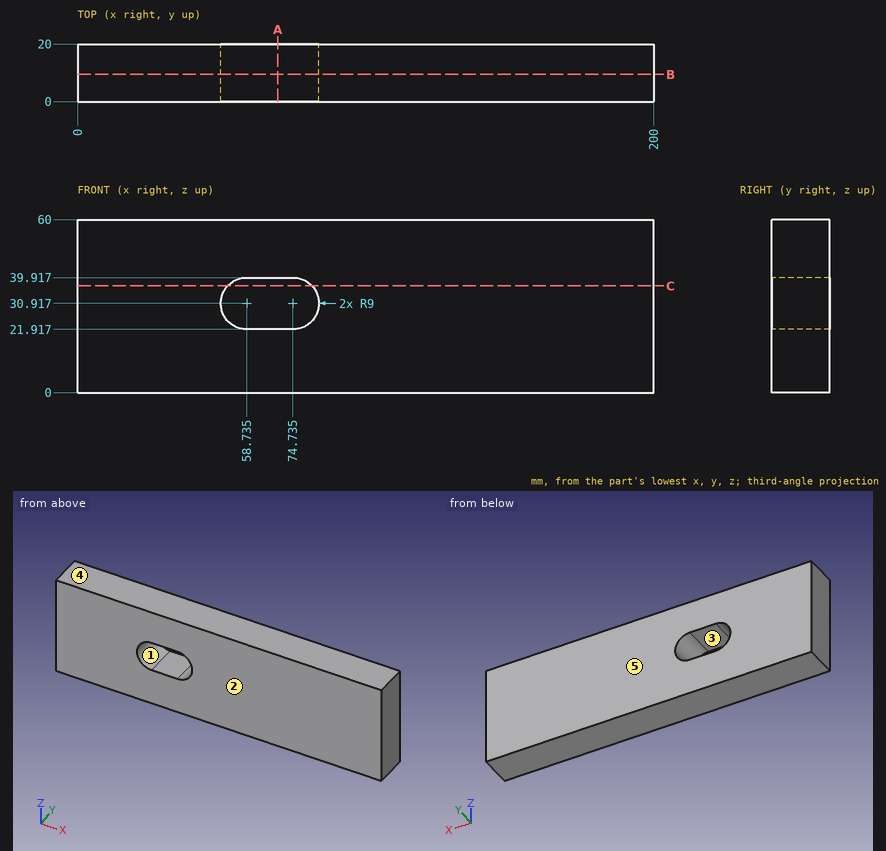
Check sheet for the drawn part. Datum: minimum x, y, z corner. Units: mm. A direction names the side the tool comes from. Coordinates: 2 decimals unless noted, no trailing zeros. Write each loop counter-clockwise with the first axis right and the second up, starting at its lowest first coordinate (ties: lowest second). Pieces come first, ordered by that corner, then holes. Notation, with made-up numbers: (45, 71.5) - (67, 71.5) arc R16 ccw to (67, 79.5) - close; hole circle Ø11 at (1, -32.5). An arc over 180 degrees is marked (long way). Answer as a JSON object with one key per item and string values.
(1) Mould release check, pull along Z, two halves, no side actions. Record for the marked faces 3, 4 and 5: pulls with the +Z half, pulls with the -Z half, needs draft (parallel to the pull), parting line crosses it, or undercut.
Report:
{"face 3": "undercut", "face 4": "pulls with the +Z half", "face 5": "needs draft"}
(2) Cross-section at C-C on z = 37. Record the cut outline in (x, y).
Report:
{"outline": "(0, 0) - (52.1, 0) - (52.1, 20) - (0, 20) - close; (81.37, 0) - (200, 0) - (200, 20) - (81.37, 20) - close"}
(3) Cross-section at B-B on y = 9.5. Record the cut outline in (x, z) (1 decimal).
Report:
{"outline": "(0, 0) - (200, 0) - (200, 60) - (0, 60) - close; hole (58.7, 21.9) - (74.7, 21.9) arc R9 ccw to (74.7, 39.9) - (58.7, 39.9) arc R9 ccw to start"}
(4) Cross-section at A-A on x = 69.5. Record the cut outline in (y, z).
Report:
{"outline": "(0, 0) - (20, 0) - (20, 21.92) - (0, 21.92) - close; (0, 39.92) - (20, 39.92) - (20, 60) - (0, 60) - close"}
(5) Thickness scan on line 1 along Z through (x, y) = (66.5, 11.5); line 2 along X through (y, z) = (18, 34); line 3 along Z through (x, y) = (80, 4.75) (1 decimal). Record the ranges inside material, lowest first.
Report:
{"line 1": "0 to 21.92, 39.92 to 60", "line 2": "0 to 50.28, 83.19 to 200", "line 3": "0 to 23.6, 38.2 to 60"}
(6) Tool access check on the marked faces 1 and 2. Record the directions out of +Z, -Z, +X, -X, +Y, -Y that give a thin tool (end or side, any length) a straight path to the whole face; none if there is none.
Report:
{"face 1": "+Y, -Y", "face 2": "+Z, -Z, +X, -X, -Y"}
